Geometry check sheet. Reference: the model listing, model coordinates, mm. A direction names the side the tool comes from. Round coordinates to 2 decimals unless told otherwise and drop trailing zeros. Order: outer loops, then holes, each group sorted by start corner. A loop starts at its lowest first (then second) coordinate and runs counter-clockwise, first axis right, second up. Notation, with made-up numbers: (-17.5, 76.25) - (-0.5, 76.25) arc R31 cw to (-0.5, 101.25) - close; hole circle Ø1 at (21.25, -8). An arc over 180 degrees is marked (long way). Use a Markdown table: item, result. Add a question column.
(1) Section check C-C on x = 1.8. Record the boundary of the cut face in (y, z), then the cut area to 3 significant figures.
(2) Section check A-A on y = 3. Record the boundary of the cut face in (x, z).
(3) Access from +Z, -Z, +X, -X, +Y, -Y to the whole of each face (thin tool, end or side, straight path). Record for faces 1 (the face through (1.233, 14.544, 2.175)), 2 (the face through (-0.27, 3.94, 1.22)).
(4) Section check B-B on y = 12.5. Record the boundary of the cut face in (x, z), then the cut area to 3 significant figures.
(5) Thickness scan on line 1 along X through (y, z) = (25.5, -0.8); line 2 along X through (y, z) = (3.5, -0.6); line 3 along Z through (x, y) = (1.8, 18.5). Record the ranges inside material, lowest first. Write a range as [from, to].
(6) Section check D-D on z = -2.1. Record the boundary of the cut face in (x, y).
(7) Mould release check, pull along X, two halves, no side actions. Record for faces 3 (the face through (-1.267, 14.544, 2.155)), 4 (the face through (0.27, 25.56, 1.22)), 5 (the face through (2.5, 15, 0)): released by +X, released by -X, zero draft, split by the parting line, or undercut.
(8) Gauge pin test, flat ends, axial feed: P1, Ø3, axis at x = 0, z = 0, coming from the -Y side (3 decimals); P2, Ø1.5, axis at y = 10.5, z = 2.5, coming from the -X side; P3, Ø3, axis at x = 0, z = 0, coming from the +Y side (3 decimals); P4, Ø2, axis at y = 26, z = 2, coming from the -X side. Record the tip position at first contact, or that the pin passes through.
```python
from build123d import *

# Parameters (mm, degrees)
BOSS_EXTRUDE1_DEPTH         = 29.5
M3_TAPPED_HOLE1_D           = 2.5
M3_TAPPED_HOLE1_DEPTH       = 7.5
M3_TAPPED_HOLE1_CSINK_D     = 3.05
M3_TAPPED_HOLE1_CSINK_ANGLE = 90
M3_TAPPED_HOLE1_TIP         = 0.751075774
M3_TAPPED_HOLE2_D           = 2.5
M3_TAPPED_HOLE2_DEPTH       = 7.5
M3_TAPPED_HOLE2_CSINK_D     = 3.05
M3_TAPPED_HOLE2_CSINK_ANGLE = 90
M3_TAPPED_HOLE2_TIP         = 0.751075774


with BuildPart() as part:
    # Sketch1 → Boss-Extrude1 (new body)
    with BuildSketch(Plane(origin=(0, 0, 0), x_dir=(1, 0, 0), z_dir=(0, 1, 0))):
        Polygon((-2.5, 1.443375673), (-2.5, -1.443375673), (0, -2.886751346), (2.5, -1.443375673), (2.5, 1.443375673), (0, 2.886751346), align=None)
    extrude(amount=BOSS_EXTRUDE1_DEPTH)

    # M3 Tapped Hole1
    with Locations(Plane(origin=(0, 29.5, 0), x_dir=(1, 0, 0), z_dir=(0, 1, 0))):
        with Locations((0, 0)):
            CounterSinkHole(M3_TAPPED_HOLE1_D / 2, M3_TAPPED_HOLE1_CSINK_D / 2, depth=M3_TAPPED_HOLE1_DEPTH, counter_sink_angle=M3_TAPPED_HOLE1_CSINK_ANGLE)
            with Locations((0, 0, -(M3_TAPPED_HOLE1_DEPTH + M3_TAPPED_HOLE1_TIP / 2))):  # 118° drill point
                Cone(0, M3_TAPPED_HOLE1_D / 2, M3_TAPPED_HOLE1_TIP, mode=Mode.SUBTRACT)

    # M3 Tapped Hole2
    with Locations(Plane(origin=(0, 0, 0), x_dir=(-1, 0, 0), z_dir=(0, -1, 0))):
        with Locations((0, 0)):
            CounterSinkHole(M3_TAPPED_HOLE2_D / 2, M3_TAPPED_HOLE2_CSINK_D / 2, depth=M3_TAPPED_HOLE2_DEPTH, counter_sink_angle=M3_TAPPED_HOLE2_CSINK_ANGLE)
            with Locations((0, 0, -(M3_TAPPED_HOLE2_DEPTH + M3_TAPPED_HOLE2_TIP / 2))):  # 118° drill point
                Cone(0, M3_TAPPED_HOLE2_D / 2, M3_TAPPED_HOLE2_TIP, mode=Mode.SUBTRACT)


solid = part.part
```
Check sheet entries:
| question | item | result |
|---|---|---|
| 1 | outline | (0, -1.85) - (29.5, -1.85) - (29.5, 1.85) - (0, 1.85) - close |
| 1 | area | 109 mm2 |
| 2 | outline | (-2.5, -1.44) - (0, -2.89) - (2.5, -1.44) - (2.5, 1.44) - (0, 2.89) - (-2.5, 1.44) - close; hole circle Ø2.5 at (0, 0) |
| 3 | face 1 | +Z, +X, +Y, -Y |
| 3 | face 2 | -Y |
| 4 | outline | (-2.5, -1.44) - (0, -2.89) - (2.5, -1.44) - (2.5, 1.44) - (0, 2.89) - (-2.5, 1.44) - close |
| 4 | area | 21.7 mm2 |
| 5 | line 1 | x = [-2.5, -0.96], [0.96, 2.5] |
| 5 | line 2 | x = [-2.5, -1.1], [1.1, 2.5] |
| 5 | line 3 | z = [-1.85, 1.85] |
| 6 | outline | (-1.36, 0) - (1.36, 0) - (1.36, 29.5) - (-1.36, 29.5) - close |
| 7 | face 3 | released by -X |
| 7 | face 4 | undercut |
| 7 | face 5 | released by +X |
| 8 | P1 | stops at y = 0.025 |
| 8 | P2 | stops at x = -1.97 |
| 8 | P3 | stops at y = 29.475 |
| 8 | P4 | stops at x = -2.5 |
